Autodesk Inventor part; units mm, degrees
ref_plane "YZ Plane" through (0, 0, 0) normal (1, 0, 0) x (0, 1, 0)
ref_plane "XY Plane" through (0, 0, 0) normal (0, 0, 1) x (1, 0, 0)
ref_plane "Upper Pickup Plane" through (0, 110, 0) normal (0, 1, 0) x (-1, 0, 0)
ref_plane "Lower Pickup Plane" through (0, -110, 0) normal (0, 1, 0) x (-1, 0, 0)
sketch "Sketch1" plane through (0, 0, 0) normal (0, 0, 1) x (1, 0, 0)
  line L0 (-70, 0) -> (70, 0) construction
  line L1 (0, 175) -> (0, -175) construction
  line L2 (30, -125) -> (-30, -125)
  line L3 (-50, -90) -> (-50, 90)
  line L4 (-30, 125) -> (30, 125)
  line L5 (50, 90) -> (50, -90)
  line L6 (-30, 125) -> (-50, 90)
  line L7 (30, 125) -> (50, 90)
  line L8 (-50, 90) -> (50, 90) construction
  line L9 (-30, -125) -> (-50, -90)
  line L10 (30, -125) -> (50, -90)
  line L11 (-50, -90) -> (50, -90) construction
  line L12 (-50, 90) -> (-50, 125) construction
  line L13 (50, 90) -> (50, 125) construction
  line L14 (-30, 125) -> (-50, 125) construction
  line L15 (30, 125) -> (50, 125) construction
  line L16 (-50, -90) -> (-50, -125) construction
  line L17 (-30, -125) -> (-50, -125) construction
  line L18 (30, -125) -> (50, -125) construction
  line L19 (50, -90) -> (50, -125) construction
  point P0 (0, 0)
  point P1 (0, 110)
  point P2 (0, -110)
  dimension "d8" = 180
  dimension "d9" = 60
  dimension "d11" = 250
  dimension "d12" = 100
extrude "Main Body" add sketch "Sketch1" along normal mid plane 30
sketch "Sketch2" plane through (0, 0, 15) normal (0, 0, 1) x (1, 0, 0)
  circle A0 centre (0, 0) radius 25
  dimension "d13" = 50
extrude "Axle Bore" cut sketch "Sketch2" against normal through all
sketch "Sketch3" plane through (0, 0, 15) normal (0, 0, 1) x (1, 0, 0)
  circle A0 centre (0, 0) radius 30
  circle A1 centre (0, 0) radius 25
  dimension "d16" = 60
extrude "Front Side Bearing Pocket" cut sketch "Sketch3" against normal blind 12
sketch "Sketch4" plane through (0, 0, -15) normal (0, 0, -1) x (-1, 0, 0)
  circle A0 centre (0, 0) radius 30
  circle A1 centre (0, 0) radius 25
extrude "Back Side Bearing Pocket" cut sketch "Sketch4" against normal blind 12
sketch "Sketch5" plane through (0, 0, 15) normal (0, 0, 1) x (1, 0, 0)
  line L0 (-50, 90) -> (-50, -90)
  line L1 (-50, -85) -> (50, -85) construction
  line L2 (50, -90) -> (50, 90)
  line L3 (0, 175) -> (0, -175) construction
  point P0 (0, 0)
  point P1 (0, -110)
  point P2 (-25, -85)
  point P3 (25, -85)
  dimension "d23" = 25
  dimension "d24" = 50
hole "Hole1" at (-25, -85, 15) at (25, -85, 15) direction (0, 0, -1) diameter 6.647 depth 30
equation "\"d4\" = Upright_Thickness"
equation "\"d13\" = Axle_Bore_Diameter"
equation "\"d16\" = Wheel_Bearing_Bore_Diameter"
equation "\"d17\" = Wheel_Bearing_Thickness"
equation "\"d19\" = Wheel_Bearing_Thickness"
equation "\"d26\" = Upright_Thickness"
equation "\"Upright_Thickness\" = 30"
equation "\"Axle_Bore_Diameter\" = 50"
equation "\"Wheel_Bearing_Bore_Diameter\" = 60"
equation "\"Wheel_Bearing_Thickness\" = 12"
equation "\"arm_z\" = 25"
properties part number "Suspension_Upright_V2"
The listing builds one solid part. Answer for the finished solid, in the listing's coordinates (mm). A direction names the side the tool comes from. Give positions to 0.01 mm unless a question says otherwise; leave off trailing zeros. Write each loop counter-clockwise with the first axis right and the second up, starting at its lowest first coordinate (ties: lowest second). Pieces come first, ordered by that corner, then holes. Notation, with made-up numbers: (32, 30) - (53, 30) arc R9 ccw to (53, 36) - close; hole circle Ø9 at (-29, 13). An arc over 180 degrees is marked (long way). One line per question, with ' | ' between items. Start each with the question number.
1. Section A-A, the plane x = 0 is taken. Determine the outline of the cut face in (y, z).
2. For faces 1 (the face through (50, 1, 0)), 2 (the face through (7, 25, -3)), 3 (the face through (-7, 25, 3)), determine the directions among +Z, -Z, +X, -X, +Y, -Y from which every point of the face is accessible in a straight line to the end or side of a thin tool.
3. Determine the mould class of faces 4 (the face through (0, -125, 0)), 5 (the face through (29.97, 1.32, -9.08)), 6 (the face through (-39.86, 107.745, -0.21)) for opening direction X: +X half, -X half, draft (parallel to the pull), parting line (faces both ways), or undercut.
4. Given P1, Ø5, axis at x = 25, y = -84.5, coming from the -Z side; P2, Ø8, axis at x = -38, z = -4.5, coming from the -Y side, each flat-ended and moving along its own axis, determine where each tip first touches the part or whether it passes through.
5. Section C-C, the plane z = 12.5 is taken. Determine the outline of the cut face in (x, y).
6. Section D-D, the plane y = -107.5 is taken. Determine the outline of the cut face in (x, z).
7. Straight lines are drawn through the part: line 1 (X direction, y = -85.5, z = -7.5); line 2 (X direction, y = -10, z = -10); line 3 (Y direction, x = 0, z = -3.25). For each, find the intervals that lie inside material, in ascending order.
8. Section B-B, the plane y = 0 is taken. Determine the outline of the cut face in (x, z), then the cut area to 3 significant figures.
Result:
1) outline: (-125, -15) - (-30, -15) - (-30, -3) - (-25, -3) - (-25, 3) - (-30, 3) - (-30, 15) - (-125, 15) - close; (25, -3) - (30, -3) - (30, -15) - (125, -15) - (125, 15) - (30, 15) - (30, 3) - (25, 3) - close
2) face 1: +Z, -Z, +X, +Y, -Y | face 2: -Z | face 3: +Z
3) face 4: draft | face 5: undercut | face 6: -X half
4) P1: passes through | P2: stops at y = -118
5) outline: (-50, -90) - (-30, -125) - (30, -125) - (50, -90) - (50, 90) - (30, 125) - (-30, 125) - (-50, 90) - close; hole circle Ø60 at (0, 0); hole circle Ø6.65 at (-25, -85); hole circle Ø6.65 at (25, -85)
6) outline: (-40, -15) - (40, -15) - (40, 15) - (-40, 15) - close
7) line 1: x = -50 to -28.29, -21.71 to 21.71, 28.29 to 50 | line 2: x = -50 to -28.28, 28.28 to 50 | line 3: y = -125 to -30, 30 to 125
8) outline: (-50, -15) - (-30, -15) - (-30, -3) - (-25, -3) - (-25, 3) - (-30, 3) - (-30, 15) - (-50, 15) - close; (25, -3) - (30, -3) - (30, -15) - (50, -15) - (50, 15) - (30, 15) - (30, 3) - (25, 3) - close | area: 1,260 mm2
